Source: three-view drawing plus pictorial views. Frame: mm from the lowest corner of the part. Give positions to 0.01 mm unless a question says otherwise; leave off trailing zeros. Order: outer loops, then holes, each group sorted by start corner. A loop starts at its lowest first (then second) coordinate and runs counter-clockwise, first axis right, second up.
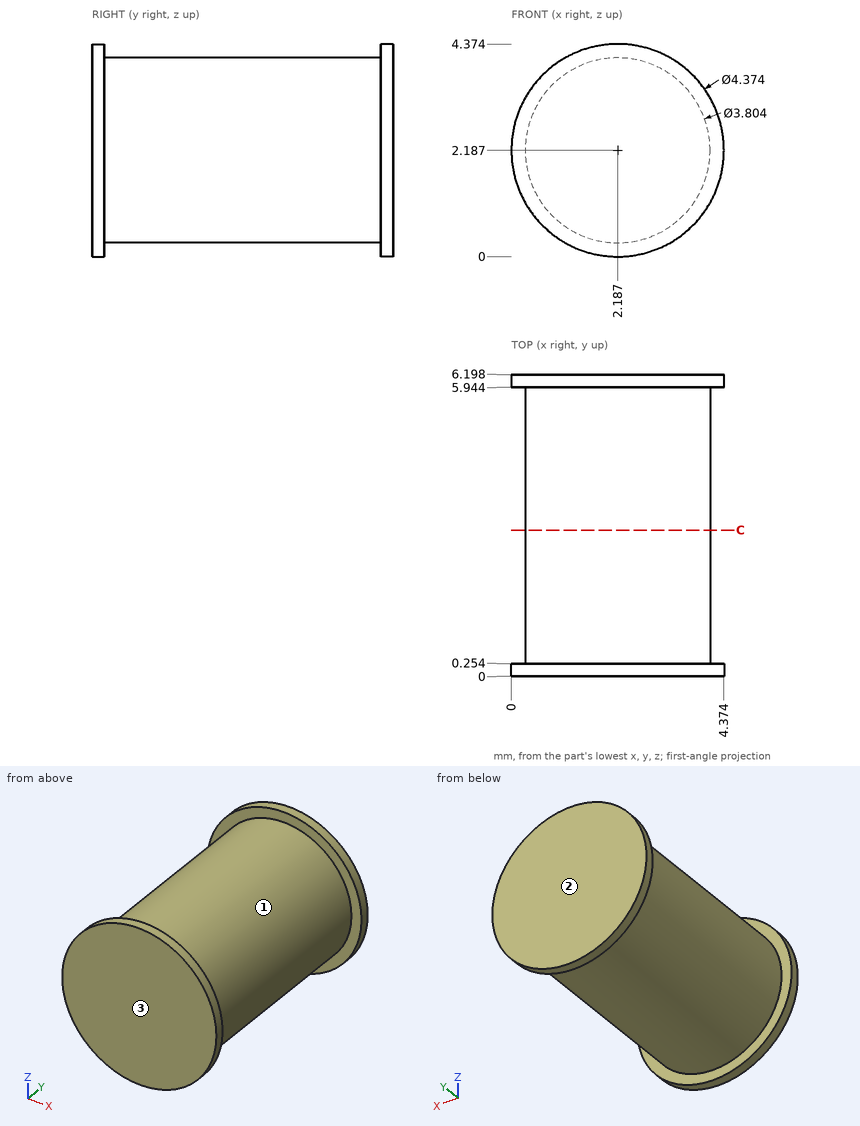
(1) Section C-C, the plane y = 3. Return loops of the section in (x, z), plus the area to 3 significant figures.
(2) Line query: line 1 along Y through (x, z) = (0.55, 3.5); line 2 along Z through (x, y) = (2.2, 0.75) (1 decimal); line 3 along X through (y, z) = (3, 3.75) (1 decimal). Output: solid intervals per line, ascending.
(3) Draft query along Y for the marked faces 1, 2 and 3. Return one class per face: +Y half, -Y half, draft (parallel to the pull), parting line (faces both ways), or undercut.
(4) Pin query (flat end, axial travel): pin 1 Ø1 at (x, y) = (3.5, 5) entering from +Z; pin 2 Ø1.5 at (x, y) = (1, 3) entering from +Z; pin 3 Ø2 at (y, z) = (4.5, 0.5) entering from -X. Return the tip coordinate at first contact, or that it passes through.
Checks:
1. outline: circle Ø3.8 at (2.19, 2.19)
1. area: 11.4 mm2
2. line 1: y = 0 to 0.25, 5.94 to 6.2
2. line 2: z = 0.3 to 4.1
2. line 3: x = 1.1 to 3.3
3. face 1: undercut
3. face 2: +Y half
3. face 3: -Y half
4. pin 1: stops at z = 3.91
4. pin 2: stops at z = 4.04
4. pin 3: stops at x = 0.41
